For this review, take the finished solid that the model builds, in its own axes (mm). A direction names the side the tool comes from. Coordinates: 2 decimals unless noted, no trailing zeros. Write each loop counter-clockwise with the first axis right and the second up, starting at its lowest first coordinate (ties: lowest second). Pieces come first, ordered by that corner, then holes. Notation, with made-up numbers: (43.25, 5.25) - (80.25, 5.25) arc R15 ccw to (80.25, 9.25) - close; hole circle Ø1 at (-36.75, 9). An arc over 180 degrees is marked (long way). Use one line per item in the form item = value. Start each with the question number.
1) We need section C-C (z = -4.5). Give the boundary of the cut face in (x, y).
2) We need section D-D (z = -19). Give the boundary of the cut face in (x, y).
3) We need section B-B (y = -8.5). Give the boundary of the cut face in (x, z), plus the area to 3 significant figures.
4) Tool access review of faces 4 (the flat face through (26.216, -5, -6)), 5 (the flat face through (-9.344, -73, -16)), 6 (the flat face through (8, -59, -30.122)), 7 (the flat face through (9, -75, -1.674)), 8 (the flat face through (9, -19, 7.978)): name each direction out of +Z, -Z, +X, -X, +Y, -Y from which nothing blocks a thin tool from reaching the whole face with its end or side.
5) For L1, parallel to X at y = -49, z = -13.5; L2, parallel to Z at x = 14, y = -47; L3, parallel to Y at x = -2, z = 2, list the stretches that pass through material, from the lowest coordinate up. Write a range as from..to.
6) Insertion check: P1, Ø14, axis at y = -59, z = -12.5, coming from the -X side; P2, Ø6, axis at x = -13.5, z = 6, coming from the -Y side; P3, Ø5.5, axis at x = 14, y = -22.5, coming from the +Z side; P4, Ø7.5, axis at y = -63.51, z = -15.9, coming from the -X side. Each pin has a flat end and moves straight along its axis. Give the tip position at first contact, or say it passes through.
7) We need section A-A (x = -8). Give the boundary of the cut face in (y, z).
8) Mouldability with a two-part tool opening along X and no side actions: class faces 1 (the flat face through (8, -10.16, -11)), 2 (the flat face through (8, -119.38, -16)), 3 (the flat face through (26.216, -75, -16)) as pulls with the +X half, pulls with the -X half, needs draft (parallel to the pull), parting line crosses it, or undercut.
```python
from build123d import *

# Parameters (mm, degrees)
F0_W      = 60.96
F0_H      = 48.26
F1_DEPTH  = 119.38
F3_DEPTH  = 130.81
F2_W      = 25.4
F2_H      = 18.288
F4_DEPTH  = 10.16
F6_DEPTH  = 12.7
F7_W      = 90.932
F7_H      = 28.448
F8_DEPTH  = 12.7
F9_W      = 90.932
F9_H      = 19.812
F10_DEPTH = 84.328
F12_DEPTH = 131.064


with BuildPart() as f1:
    # F0 (on Front) → F1 (new body)
    with BuildSketch(Plane.XZ):
        with Locations((8.435591, -5.991532)):
            Rectangle(F0_W, F0_H)
    extrude(amount=F1_DEPTH)

    # F2 (on face) → F3 (cut)
    with BuildSketch(Plane.XY.offset(18.138468)):
        Polygon((26.215591, 0), (-9.344409, 0), (-9.344409, -10.16), (-3.902869, -10.16), (21.497131, -10.16), (26.215591, -10.16), align=None)
    extrude(amount=-F3_DEPTH, mode=Mode.SUBTRACT)

    # F2 (on face) → F4 (cut)
    with BuildSketch(Plane.XY.offset(18.138468)):
        with Locations((8.797131, -19.304)):
            Rectangle(F2_W, F2_H)
    extrude(amount=-F4_DEPTH, mode=Mode.SUBTRACT)

    # F5 (on face) → F6 (cut)
    with BuildSketch(Plane(origin=(-22.044409, 0, 0), x_dir=(0, -1, 0), z_dir=(-1, 0, 0))):
        Polygon((28.448, -1.673532), (28.448, -30.121532), (142.968658, -30.121532), (142.526776, 0), align=None)
    extrude(amount=-F6_DEPTH, mode=Mode.SUBTRACT)

    # F7 (on face) → F8 (cut)
    with BuildSketch(Plane.YZ.offset(38.915591)):
        with Locations((-73.914, -15.897532)):
            Rectangle(F7_W, F7_H)
    extrude(amount=-F8_DEPTH, mode=Mode.SUBTRACT)

    # F9 (on face) → F10 (cut)
    with BuildSketch(Plane.YZ.offset(38.915591)):
        with Locations((-73.914, 8.232468)):
            Rectangle(F9_W, F9_H)
    extrude(amount=-F10_DEPTH, mode=Mode.SUBTRACT)

    # F11 (on face) → F12 (cut)
    with BuildSketch(Plane(origin=(-9.344409, 0, 0), x_dir=(0, -1, 0), z_dir=(-1, 0, 0))):
        with BuildLine():
            ThreePointArc((63.508675, -22.247532), (67.998803, -20.387661), (69.858675, -15.897532))
            ThreePointArc((69.858675, -15.897532), (59.018546, -11.407404), (63.508675, -22.247532))
        make_face()
    extrude(amount=-F12_DEPTH, mode=Mode.SUBTRACT)


solid = f1.part
```
Determined:
q1.outline = (-22.04, -28.45) - (-9.34, -28.45) - (-9.34, -119.38) - (26.22, -119.38) - (26.22, -28.45) - (38.92, -28.45) - (38.92, 0) - (26.22, 0) - (26.22, -10.16) - (-9.34, -10.16) - (-9.34, 0) - (-22.04, 0) - close
q2.outline = (-22.04, -28.45) - (-9.34, -28.45) - (-9.34, -57.97) - (26.22, -57.97) - (26.22, -28.45) - (38.92, -28.45) - (38.92, 0) - (26.22, 0) - (26.22, -10.16) - (-9.34, -10.16) - (-9.34, 0) - (-22.04, 0) - close; (-9.34, -119.38) - (26.22, -119.38) - (26.22, -69.05) - (-9.34, -69.05) - close
q3.outline = (-22.04, -30.12) - (-9.34, -30.12) - (-9.34, 18.14) - (-22.04, 18.14) - close; (26.22, -30.12) - (38.92, -30.12) - (38.92, 18.14) - (26.22, 18.14) - close
q3.area = 1,230 mm²
q4.face_4 = +Z, -Z, +Y
q4.face_5 = +Z, -Z, -X, -Y
q4.face_6 = -Z, +X, -X, +Y, -Y
q4.face_7 = +Z, +X, -X, -Y
q4.face_8 = +Z, +Y, -Y
q5.L1 = -9.34..26.22
q5.L2 = -30.12..-1.67
q5.L3 = -28.45..-10.16
q6.P1 = -9.34
q6.P2 = -28.45
q6.P3 = 7.98
q6.P4 = through
q7.outline = (-119.38, -30.12) - (-10.16, -30.12) - (-10.16, 18.14) - (-28.45, 18.14) - (-28.45, -1.67) - (-119.38, -1.67) - close; hole (-69.86, -15.9) arc R6.35 ccw to (-63.51, -22.25) arc R6.35 ccw (long way) to start
q8.face_1 = undercut
q8.face_2 = needs draft
q8.face_3 = pulls with the +X half
